Input: part model. Units: mm. Frame: model coordinates. A direction names the side the tool comes from. Give positions to 0.01 mm unless a question says otherwise; leave off trailing zeros. Loops run counter-clockwise (first coordinate to the right, second up) from the corner with the lowest first, then second, coordinate; pieces in that order, holes last. Notation, with made-up numbers: (-36, 80.5) - (-29, 80.5) arc R27 ccw to (-29, 96.5) - close; hole circle Ø3 at (61, 84.5). An arc over 180 degrees is marked (long way). Answer as a JSON object with one key per item and string values.
from build123d import *

# Parameters (mm, degrees)
SKETCH1_R               = 3.175
BOSS_EXTRUDE1_DEPTH     = 22.225
CUT_EXTRUDE1_DEPTH      = 1
CUT_EXTRUDE1_DEPTH_BACK = 9.525
CHAMFER1_SIZE           = 1


with BuildPart() as part:
    # Sketch1 → Boss-Extrude1 (new body)
    with BuildSketch(Plane.XY):
        Circle(SKETCH1_R)
    extrude(amount=BOSS_EXTRUDE1_DEPTH)

    # Sketch3 → Cut-Extrude1 (cut, two sides)
    with BuildSketch(Plane.XY.offset(22.225)) as cut_extrude1_sk:
        Polygon((-27.877607345, 0.7874), (-3.075813102, 0.7874), (3.075813102, 0.7874), (27.877607345, 0.7874), (27.877607345, 50.390988485), (-27.877607345, 50.390988485), align=None)
    extrude(amount=CUT_EXTRUDE1_DEPTH, mode=Mode.SUBTRACT)
    extrude(cut_extrude1_sk.sketch, amount=-CUT_EXTRUDE1_DEPTH_BACK, mode=Mode.SUBTRACT)

    # Chamfer1
    chamfer1_edges = [part.edges().sort_by_distance(p)[0] for p in [
        (-0.39681129, -3.150105681, 22.225),
    ]]
    chamfer(chamfer1_edges, length=CHAMFER1_SIZE)


solid = part.part
Item 1: Access query for faces 1 (the face through (0, 0, 22.225)), 2 (the face through (0, 2, 12.7)). Directions: +Z, -Z, +X, -X, +Y, -Y. A direction counts if a zero-diameter tool reaches every point of the face in a straight line with its end or side. Return the directions, or none.
Geometry check:
{"face 1": "+Z, +X, -X, +Y, -Y", "face 2": "+Z, +X, -X, +Y"}
Item 2: Cut plane C-C (y = 2.5). Return loops of the section in (x, z), then the cut area to 3 significant figures.
Geometry check:
{"outline": "(-1.96, 0) - (1.96, 0) - (1.96, 12.7) - (-1.96, 12.7) - close", "area": "49.7 mm2"}
Item 3: Contact query for flat-ended pins moving along their axis: P1, Ø2, axis at x = -2.5, z = 13, coming from the +Y side; P2, Ø2.5, axis at x = -1, y = 1.5, coming from the +Z side (3 decimals); P3, Ø1.8, axis at x = 1, z = 18.5, coming from the +Y side. Output: stop coordinate, or through.
Geometry check:
{"P1": "stops at y = 2.77", "P2": "stops at z = 22.225", "P3": "stops at y = 0.79"}
Item 4: Cut plane A-A (x = 0). Return loops of the section in (y, z) (3 decimals).
Geometry check:
{"outline": "(-3.175, 0) - (3.175, 0) - (3.175, 12.7) - (0.787, 12.7) - (0.787, 22.225) - (-2.175, 22.225) - (-3.175, 21.225) - close"}
Item 5: Cut plane B-B (z = 7.5). Return loops of the section in (x, y) (3 decimals).
Geometry check:
{"outline": "circle Ø6.35 at (0, 0)"}
Item 6: Material intervals for line 1 (Z direction, x = -0.75, y = 1); line 2 (X direction, y = -1, z = 18); line 3 (X direction, y = 2.5, z = 4.75), sorted ascending. Write a range as [from, to].
Geometry check:
{"line 1": "z = [0, 12.7]", "line 2": "x = [-3.01, 3.01]", "line 3": "x = [-1.96, 1.96]"}
